```python
from build123d import *

# Parameters (mm, degrees)
BOSS_EXTRUDE1_DEPTH = 90
FILLET1_R           = 1
SKETCH2_R           = 15
CUT_EXTRUDE1_DEPTH  = 10


with BuildPart() as part:
    # Sketch1 → Boss-Extrude1 (new body)
    with BuildSketch(Plane.XY):
        Polygon((-20, -2.032342801), (-20, -10), (20, -10), (20, -2.032342801), (17, 10), (-17, 10), align=None)
    extrude(amount=BOSS_EXTRUDE1_DEPTH)

    # Fillet1
    fillet1_edges = [part.edges().sort_by_distance(p)[0] for p in [
        (17, 10, 45),
        (20, -2.032342801, 45),
        (20, -10, 45),
        (-20, -10, 45),
        (-20, -2.032342801, 45),
        (-17, 10, 45),
    ]]
    fillet(fillet1_edges, radius=FILLET1_R)

    # Sketch2 → Cut-Extrude1 (cut)
    with BuildSketch(Plane(origin=(0, 10, 0), x_dir=(1, 0, 0), z_dir=(0, 1, 0))):
        with Locations(Location((0, -45.17837191, 0), (0, 0, 270))):
            Circle(SKETCH2_R)
    extrude(amount=-CUT_EXTRUDE1_DEPTH, mode=Mode.SUBTRACT)


solid = part.part
```
Geometry check sheet. Reference: the model listing, model coordinates, mm. A direction names the side the tool comes from. Give positions to 0.01 mm unless a question says otherwise; leave off trailing zeros. Order: outer loops, then holes, each group sorted by start corner. A loop starts at its lowest first (then second) coordinate and runs counter-clockwise, first axis right, second up. Notation, with made-up numbers: (56, 10) - (65, 10) arc R28 cw to (65, 31) - close; hole circle Ø6 at (-13.75, 74). An arc over 180 degrees is marked (long way). Answer in a Markdown table with one row per item. Add a question column.
Q1. Material ranges on probe 1 along Y at (x, z) = (-7.5, 57); probe 2 along X at (y, z) = (-2, 76); probe 3 along Z at (x, y) = (-13, 7), recorded low to high. Write a range as from..to.
Q2. Cross-section at D-D, the plane z = 35.5. Enter the section's corners in (x, y).
Q3. Mould release check, pull along X, two halves, no side actions. Record for faces 1 (the flat face through (0, -10, 44)), 2 (the flat face through (0, 0, 45)), 3 (the flat face through (18.6, 3.59, 44.37)): pulls with the +X half, pulls with the -X half, needs draft (parallel to the pull), parting line crosses it, or undercut.
Q4. Tool access check on faces 4 (the cylindrical face through (-5.745, 5.07, 59.035)), 5 (the flat face through (-18.56, 3.74, 44.37)). Record the directions out of +Z, -Z, +X, -X, +Y, -Y that give a thin tool (end or side, any length) a straight path to the whole face; none if there is none.
Q5. Cross-section at A-A, the plane z = 25. Enter the section's corners in (x, y).
Q6. Gauge pin test, flat ends, axial feed: pin 1 (1 mm diameter, centred on y = 3.5, z = 14, fed in from -X); pin 2 (6 mm diameter, centred on y = 1, z = 80.5, fed in from +X); pin 3 (9 mm diameter, centred on x = 3, z = 43.5, fed in from +Y). Record the tip position at first contact, or that the pin passes through.
Q7. Cross-section at C-C, the plane y = 7. Enter the section's corners in (x, z), then the cut area to 3 significant figures.
Q8. Cross-section at B-B, the plane x = 0. Enter the section's corners in (y, z).
Check values:
| question | item | result |
|---|---|---|
| 1 | probe 1 | y = -10..0 |
| 1 | probe 2 | x = -19.99..19.99 |
| 1 | probe 3 | z = 0..37.7, 52.66..90 |
| 2 | outline | (-20, -9) arc R1 ccw to (-19, -10) - (19, -10) arc R1 ccw to (20, -9) - (20, -2.16) arc R1 ccw to (19.97, -1.91) - (17.19, 9.24) arc R1 ccw to (16.22, 10) - (11.46, 10) - (11.46, 0) - (-11.46, 0) - (-11.46, 10) - (-16.22, 10) arc R1 ccw to (-17.19, 9.24) - (-19.97, -1.91) arc R1 ccw to (-20, -2.16) - close |
| 3 | face 1 | needs draft |
| 3 | face 2 | undercut |
| 3 | face 3 | pulls with the +X half |
| 4 | face 4 | +Y |
| 4 | face 5 | +Z, -Z, -X, +Y |
| 5 | outline | (-20, -9) arc R1 ccw to (-19, -10) - (19, -10) arc R1 ccw to (20, -9) - (20, -2.16) arc R1 ccw to (19.97, -1.91) - (17.19, 9.24) arc R1 ccw to (16.22, 10) - (-16.22, 10) arc R1 ccw to (-17.19, 9.24) - (-19.97, -1.91) arc R1 ccw to (-20, -2.16) - close |
| 6 | pin 1 | stops at x = -18.75 |
| 6 | pin 2 | stops at x = 19.99 |
| 6 | pin 3 | stops at y = 0 |
| 7 | outline | (-17.75, 0) - (17.75, 0) - (17.75, 90) - (-17.75, 90) - close; hole circle Ø30 at (0, 45.18) |
| 7 | area | 2,490 mm^2 |
| 8 | outline | (-10, 0) - (10, 0) - (10, 30.18) - (0, 30.18) - (0, 60.18) - (10, 60.18) - (10, 90) - (-10, 90) - close |
